```python
from build123d import *

# Parameters (mm, degrees)
F0_W     = 668
F0_H     = 500
F1_DEPTH = 12


with BuildPart() as f1:
    # F0 (on Front) → F1 (new body)
    with BuildSketch(Plane.XZ):
        with Locations((334, 250)):
            Rectangle(F0_W, F0_H)
        with BuildLine():
            Line((140, 140), (125, 140))
            ThreePointArc((125, 140), (75.502525, 160.502525), (55, 210))
            Line((55, 210), (55, 290))
            ThreePointArc((55, 290), (75.502525, 339.497475), (125, 360))
            Line((125, 360), (140, 360))
            ThreePointArc((140, 360), (189.497475, 339.497475), (210, 290))
            Line((210, 290), (210, 210))
            ThreePointArc((210, 210), (189.497475, 160.502525), (140, 140))
        make_face(mode=Mode.SUBTRACT)
        with BuildLine():
            Line((543, 140), (528, 140))
            ThreePointArc((528, 140), (478.502525, 160.502525), (458, 210))
            Line((458, 210), (458, 290))
            ThreePointArc((458, 290), (478.502525, 339.497475), (528, 360))
            Line((528, 360), (543, 360))
            ThreePointArc((543, 360), (592.497475, 339.497475), (613, 290))
            Line((613, 290), (613, 210))
            ThreePointArc((613, 210), (592.497475, 160.502525), (543, 140))
        make_face(mode=Mode.SUBTRACT)
    extrude(amount=F1_DEPTH)


solid = f1.part
```
The listing builds one solid part. Answer for the finished solid, in the listing's coordinates (mm). A direction names the side the tool comes from. Round coordinates to 2 decimals unless told otherwise and drop trailing zeros. Loops run counter-clockwise (first coordinate to the right, second up) from the corner with the lowest first, then second, coordinate; pieces in that order, holes last. Notation, with made-up numbers: (4.5, 17.5) -> (35.5, 17.5) arc R19 cw to (35.5, 26.5) -> close; hole circle Ø5 at (-39, 74). An arc over 180 degrees is marked (long way). Use one line per item in the form item = value.
1. For a pull along X with two mould halves and no side action, classify faces 1 (the flat face through (329, 0, 254)), 2 (the cylindrical face through (593.04, -5.92, 161.05)), 3 (the cylindrical face through (591.95, -5.92, 340.04)) as released by +X, released by -X, zero draft, split by the parting line, or undercut.
Answer key:
face_1 = zero draft
face_2 = undercut
face_3 = undercut
2. The part is cut by section A-A on z = 271. Determine the outline of the cut face in (x, y), and give its area (3 significant figures).
Answer key:
outline = (0, -12) -> (55, -12) -> (55, 0) -> (0, 0) -> close; (210, -12) -> (458, -12) -> (458, 0) -> (210, 0) -> close; (613, -12) -> (668, -12) -> (668, 0) -> (613, 0) -> close
area = 4,300 mm²
3. The part is cut by section C-C on x = 535. Determine the outline of the cut face in (y, z), and give its area (3 significant figures).
Answer key:
outline = (-12, 0) -> (0, 0) -> (0, 140) -> (-12, 140) -> close; (-12, 360) -> (0, 360) -> (0, 500) -> (-12, 500) -> close
area = 3,360 mm²
4. A tool of negligible diameter and unlimited length cuts with its end or side. For faces 4 (the cylindrical face through (74.96, -5.92, 338.95)), 5 (the flat face through (329, -12, 254)), from which of +Z, -Z, +X, -X, +Y, -Y can it reach the whole face along a straight path? Write none if from no direction.
Answer key:
face_4 = +Y, -Y
face_5 = +Z, -Z, +X, -X, -Y
5. The part is cut by section D-D on x = 166.5. Determine the outline of the cut face in (y, z), and give its area (3 significant figures).
Answer key:
outline = (-12, 0) -> (0, 0) -> (0, 145.21) -> (-12, 145.21) -> close; (-12, 354.79) -> (0, 354.79) -> (0, 500) -> (-12, 500) -> close
area = 3,490 mm²
6. The part is cut by section B-B on y = -8. Determine the outline of the cut face in (x, z).
Answer key:
outline = (0, 0) -> (668, 0) -> (668, 500) -> (0, 500) -> close; hole (55, 210) arc R70 ccw to (125, 140) -> (140, 140) arc R70 ccw to (210, 210) -> (210, 290) arc R70 ccw to (140, 360) -> (125, 360) arc R70 ccw to (55, 290) -> close; hole (458, 210) arc R70 ccw to (528, 140) -> (543, 140) arc R70 ccw to (613, 210) -> (613, 290) arc R70 ccw to (543, 360) -> (528, 360) arc R70 ccw to (458, 290) -> close
7. Find the intervals of material crossed by probe 1 along X at (y, z) = (-6.25, 212); probe 2 along X at (y, z) = (-5.5, 178); probe 3 along Z at (x, y) = (102, -8), in increasing order. Write a range as [from, to].
Answer key:
probe_1 = [0, 55], [210, 458], [613, 668]
probe_2 = [0, 62.74], [202.26, 465.74], [605.26, 668]
probe_3 = [0, 143.89], [356.11, 500]
8. A flat-ended cylindrical pin translates along its axis: pin 1 Ø6 at (x, y) = (538.5, -3.5) entering from -Z. Find the tip coordinate at first contact, or state that the pin passes through.
Answer key:
pin_1 = 0
